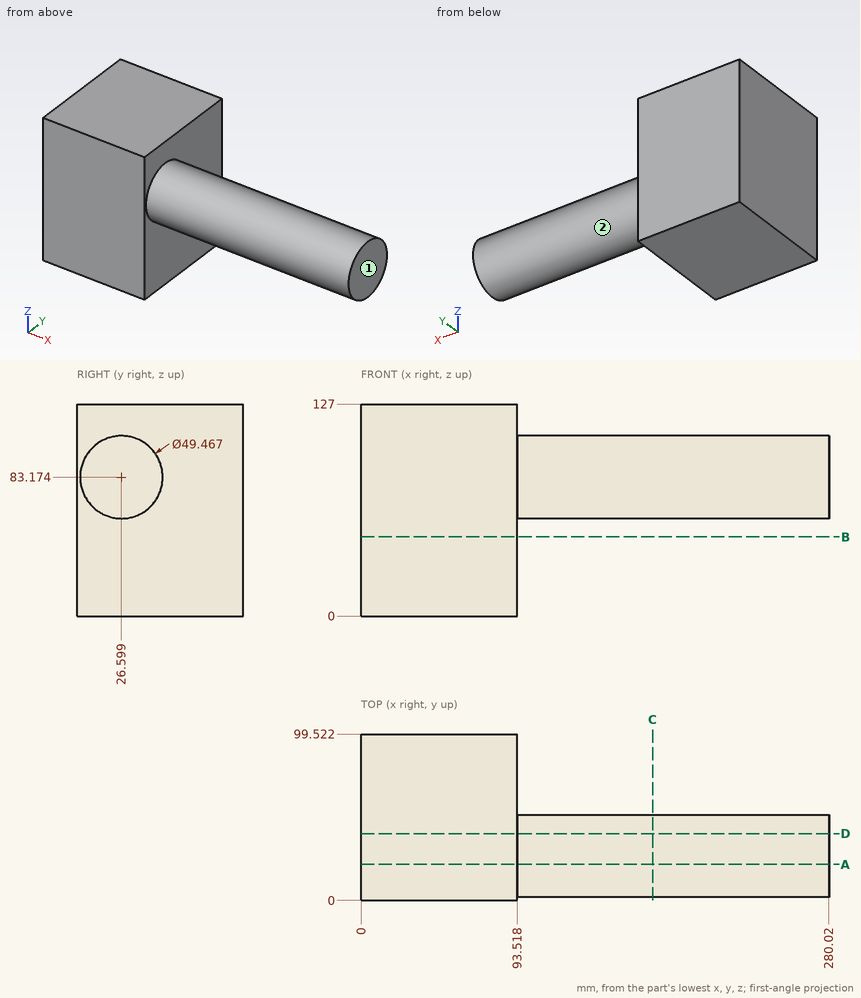
Here's the drawing with two shaded views (mm, measured from the low corner). I have some questions. A direction names the side the tool comes from. Coordinates: 2 decimals unless noted, no trailing zeros. Order: outer loops, then holes, each group sorted by start corner. A loop starts at its lowest first (then second) coordinate and runs counter-clockwise, first axis right, second up.
Item 1: I need wall thicknesses on probe 1 along X at (y, z) = (42, 41.5); probe 2 along Z at (x, y) = (231, 19); probe 3 along Y at (x, z) = (100, 96). Which ranges of each line are inside material? Lowest first, please.
Response values:
probe 1: x = 0 to 93.52
probe 2: z = 59.64 to 106.71
probe 3: y = 5.45 to 47.75
Item 2: If we section it at B-B, the plane z = 47.5: List the corners of the cut face in (x, y) for me, then the cut area to 3 significant figures.
Response values:
outline: (0, 0) - (93.52, 0) - (93.52, 99.52) - (0, 99.52) - close
area: 9,310 mm2
Item 3: I'm going to push flat-ended pins straight in: pin 1 Ø10 at (x, y) = (205.5, 19.5) entering from -Z; pin 2 Ø10 at (x, z) = (224, 97) entering from +Y (1 decimal); pin 3 Ø12 at (y, z) = (78.5, 109.5) entering from +X. Where does each tip first touch, or does it pass through?
Response values:
pin 1: stops at z = 58.53
pin 2: stops at y = 49.7
pin 3: stops at x = 93.52
Item 4: If we section it at A-A, the plane y = 21.5: List the corners of the cut face in (x, z) for me, then the cut area to 3 significant figures.
Response values:
outline: (0, 0) - (93.52, 0) - (93.52, 58.97) - (280.02, 58.97) - (280.02, 107.38) - (93.52, 107.38) - (93.52, 127) - (0, 127) - close
area: 20,900 mm2
Item 5: If we section it at C-C, the plane x = 174.5: List the corners of the cut face in (y, z) for me (1 decimal), then the cut area to 3 significant figures.
Response values:
outline: circle Ø49.5 at (26.6, 83.2)
area: 1,920 mm2
Item 6: If we section it at D-D, the plane y = 40: List the corners of the cut face in (x, z) for me (1 decimal), then the cut area to 3 significant figures.
Response values:
outline: (0, 0) - (93.5, 0) - (93.5, 62.4) - (280, 62.4) - (280, 104) - (93.5, 104) - (93.5, 127) - (0, 127) - close
area: 19,600 mm2
Item 7: Which directions (+Z, -Z, +X, -X, +Y, -Y) give clear straight access to the entire face, cutting with the end or side of a thin tool? Please do the marked faces 1 and 2.
Response values:
face 1: +Z, -Z, +X, +Y, -Y
face 2: +X
